Source: three-view drawing plus pictorial views. Frame: mm from the lowest corner of the part. A direction names the side the tool comes from. Give positions to 0.01 mm unless a question says otherwise; leave off trailing zeros. Order: outer loops, then holes, each group sorted by start corner. A loop starts at its lowest first (then second) coordinate and runs counter-clockwise, first axis right, second up. Notation, with made-up numbers: (-8.75, 29.25) - (46.25, 29.25) arc R16 cw to (46.25, 46.25) - close; hole circle Ø4 at (23, 45.5). An arc over 180 degrees is marked (long way). Answer in a Markdown table with one row per item. Add a question column.
1. Ray query, line 1 (X direction, y = 11.75, z = 3.5); line 2 (X direction, y = 12.5, z = 5.25); line 3 (Z direction, x = 43, y = 5). Return the intervals inside material, ascending. Write a range as [from, to].
2. Mould query, pull axis X, two halves, no side actions, for the marked faces 1, 2, 3 and 4. Classes: released by +X, released by -X, zero draft, split by the parting line, or undercut.
3. Section query B-B on x = 24.4. Return loops of the section in (y, z).
4. Section query D-D on y = 15. Return loops of the section in (x, z), and give its area (3 significant figures).
5. Access query for the marked faces 5, 6 and 7. Directions: +Z, -Z, +X, -X, +Y, -Y. A direction counts if a zero-diameter tool reaches every point of the face in a straight line with its end or side. Return the directions, or none.
6. Section query C-C on z = 4.25. Count the separate pieces of the cut face and the enclosed holes in it, and give its area (3 significant figures).
7. Contact query for flat-ended pins moving along their axis: pin 1 (4 mm diameter, centred on x = 40, z = 5, fed in from -Y); pin 2 (3 mm diameter, centred on x = 21, y = 11.5, fed in from +Z). Output: stop coordinate, or through.
8. Section query A-A on y = 5. Return loops of the section in (x, z).
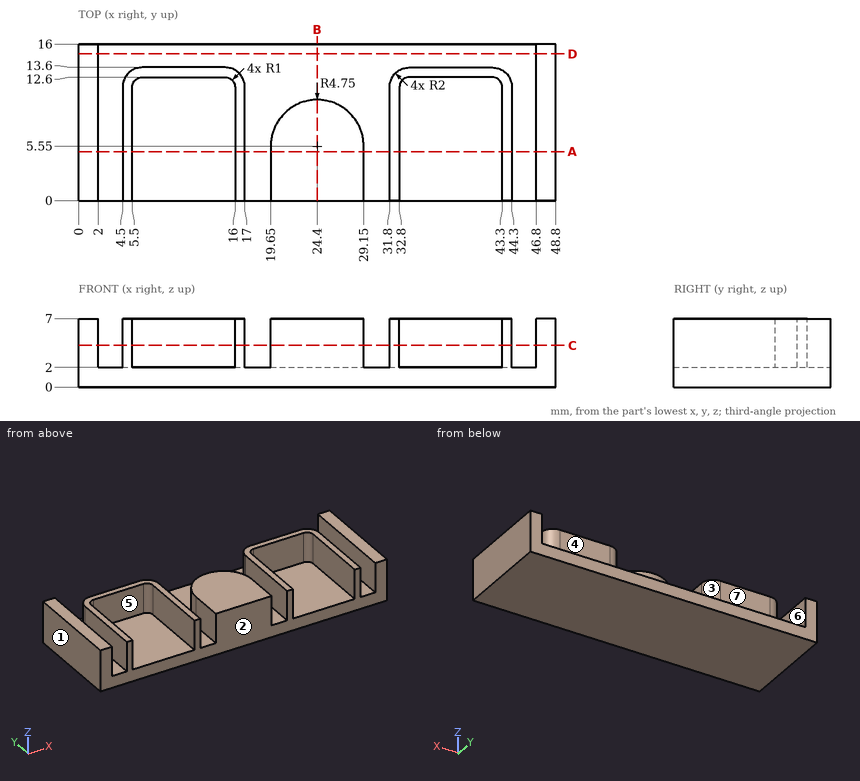
Answer:
| question | item | result |
|---|---|---|
| 1 | line 1 | x = [0, 2], [4.51, 5.51], [15.99, 16.99], [31.81, 32.81], [43.29, 44.29], [46.8, 48.8] |
| 1 | line 2 | x = [0, 2], [4.71, 6.06], [15.44, 16.79], [32.01, 33.36], [42.74, 44.09], [46.8, 48.8] |
| 1 | line 3 | z = [0, 2] |
| 2 | face 1 | released by -X |
| 2 | face 2 | zero draft |
| 2 | face 3 | undercut |
| 2 | face 4 | undercut |
| 3 | outline | (0, 0) - (16, 0) - (16, 2) - (10.3, 2) - (10.3, 7) - (0, 7) - close |
| 4 | outline | (0, 0) - (48.8, 0) - (48.8, 7) - (46.8, 7) - (46.8, 2) - (2, 2) - (2, 7) - (0, 7) - close |
| 4 | area | 118 mm² |
| 5 | face 5 | +Z, -Y |
| 5 | face 6 | +Z, +Y, -Y |
| 5 | face 7 | +Z, +Y |
| 6 | separate pieces | 5 |
| 6 | enclosed holes | 0 |
| 6 | area | 225 mm² |
| 7 | pin 1 | stops at y = 12.6 |
| 7 | pin 2 | stops at z = 2 |
| 8 | outline | (0, 0) - (48.8, 0) - (48.8, 7) - (46.8, 7) - (46.8, 2) - (44.3, 2) - (44.3, 7) - (43.3, 7) - (43.3, 2) - (32.8, 2) - (32.8, 7) - (31.8, 7) - (31.8, 2) - (29.15, 2) - (29.15, 7) - (19.65, 7) - (19.65, 2) - (17, 2) - (17, 7) - (16, 7) - (16, 2) - (5.5, 2) - (5.5, 7) - (4.5, 7) - (4.5, 2) - (2, 2) - (2, 7) - (0, 7) - close |
